Source: CAD feature listing. Evaluate the final solid. Frame: model axes, mm. Face numbers are marked on the shaded views. Round coordinates to 2 decimals unless told otherwise and drop trailing zeros. Order: outer loops, then holes, each group sorted by start corner. A loop starts at its lowest first (then second) coordinate and runs counter-clockwise, first axis right, second up. Notation, with made-up numbers: (4.5, 15.25) -> (43.5, 15.25) arc R18 cw to (43.5, 35.25) -> close; hole circle Ø3 at (75, 64.5). An arc over 180 degrees is marked (long way). Answer as CSV lines item,"result". Start each with the question number.
(1) Section query B-B (y = -31). Output: boundary loops of the cut face in (x, z), plus the area to 3 significant figures.
(2) Section query D-D (y = -88). Output: boundary loops of the cut face in (x, z), plus the area to 3 significant figures.
(3) Section query A-A (x = -3.5). Output: boundary loops of the cut face in (y, z).
(4) Contact query for flat-ended pins moving along their axis: P1, Ø1, axis at y = -51, z = 2.5, coming from the +X side; P2, Ø1, axis at x = 2.5, z = 0.5, coming from the +Y side; P3, Ø2, axis at y = -26.5, z = 3, coming from the -X side. Output: stop coordinate, or through.
(5) Section query C-C (z = 2). Output: boundary loops of the cut face in (x, y).
(6) Pull-direction query (Z, two-part tool) for the marked faces 1 and 2; classes: +Z half, -Z half, draft (parallel to the pull), parting line (faces both ways), or undercut.
(7) Line query: line 1 along X through (y, z) = (-68, 3.4); line 2 along Y through (x, z) = (-16, 3.2); line 3 along X through (y, z) = (-118, 0.25). Output: solid intervals per line, ascending. Write a range as from..to.
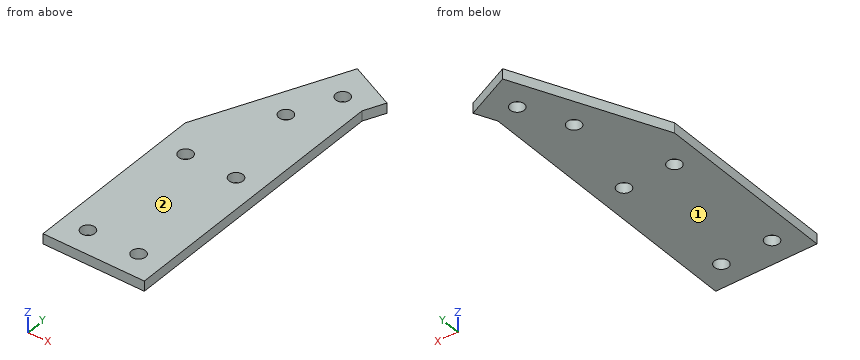
```python
from build123d import *

# Parameters (mm, degrees)
BOSS_EXTRUDE1_DEPTH = 4
SKETCH2_R           = 2.75
CUT_EXTRUDE1_DEPTH  = 4
SKETCH3_R           = 2.75
CUT_EXTRUDE2_DEPTH  = 4


with BuildPart() as part:
    # Sketch1 → Boss-Extrude1 (new body)
    with BuildSketch(Plane.XY):
        Polygon((0, 0), (18.168649127, -8.360633284), (14.494150799, -16.345754575), (14.688182734, -127.505585232), (-25.311817266, -127.505585232), (-25.311817266, -55.005585232), align=None)
    extrude(amount=BOSS_EXTRUDE1_DEPTH)

    # Sketch2 → Cut-Extrude1 (cut)
    with BuildSketch(Plane.XY.offset(4)):
        with Locations((-15.311817266, -117.505585232)):
            Circle(SKETCH2_R)
        with Locations((4.670712279, -117.505585232)):
            Circle(SKETCH2_R)
        with Locations((-15.311817266, -67.755585232)):
            Circle(SKETCH2_R)
        with Locations((4.583872557, -67.755585232)):
            Circle(SKETCH2_R)
    extrude(amount=-CUT_EXTRUDE1_DEPTH, mode=Mode.SUBTRACT)

    # Sketch3 → Cut-Extrude2 (cut)
    with BuildSketch(Plane.XY.offset(4)):
        with Locations((5.271808516, -14.259489296)):
            Circle(SKETCH3_R)
        with Locations((-3.088824768, -32.428138423)):
            Circle(SKETCH3_R)
    extrude(amount=-CUT_EXTRUDE2_DEPTH, mode=Mode.SUBTRACT)


solid = part.part
```
Answer block:
1,outline,"(-14.27, 0) -> (-5.44, 0) -> (-5.44, 4) -> (-14.27, 4) -> close; (-0.74, 0) -> (14.52, 0) -> (14.52, 4) -> (-0.74, 4) -> close"
1,area,"96.3 mm2"
2,outline,"(-25.31, 0) -> (14.62, 0) -> (14.62, 4) -> (-25.31, 4) -> close"
2,area,"160 mm2"
3,outline,"(-127.51, 0) -> (-35.15, 0) -> (-35.15, 4) -> (-127.51, 4) -> close; (-29.71, 0) -> (-7.61, 0) -> (-7.61, 4) -> (-29.71, 4) -> close"
4,P1,"x = 14.56"
4,P2,"y = -0.92"
4,P3,"x = -12.65"
5,outline,"(-25.31, -127.51) -> (14.69, -127.51) -> (14.49, -16.35) -> (18.17, -8.36) -> (0, 0) -> (-25.31, -55.01) -> close; hole circle Ø5.5 at (-15.31, -117.51); hole circle Ø5.5 at (-15.31, -67.76); hole circle Ø5.5 at (-3.09, -32.43); hole circle Ø5.5 at (4.58, -67.76); hole circle Ø5.5 at (4.67, -117.51); hole circle Ø5.5 at (5.27, -14.26)"
6,face 1,"-Z half"
6,face 2,"+Z half"
7,line 1,"-25.31..-18.05, -12.57..1.84, 7.32..14.58"
7,line 2,"-127.51..-120.17, -114.84..-70.42, -65.09..-34.77"
7,line 3,"-25.31..-18.02, -12.61..1.97, 7.38..14.67"
